Source: CAD feature listing. Evaluate the final solid. Frame: model axes, mm. Face numbers are marked on the shaded views. A direction names the side the tool comes from. Give positions to 0.01 mm unless a question says otherwise; leave off trailing zeros. Write each loop counter-clockwise with the first axis right and the second up, starting at its lowest first coordinate (ties: lowest second). Pieces come first, ordered by that corner, then holes. Notation, with made-up numbers: M 84.25,47.5 L 128.25,47.5 A15 ccw 128.25,71.5 Z; hole C -18.75,24 d11. An arc over 180 degrees is marked long. Return JSON: item names as keys, results as strings.
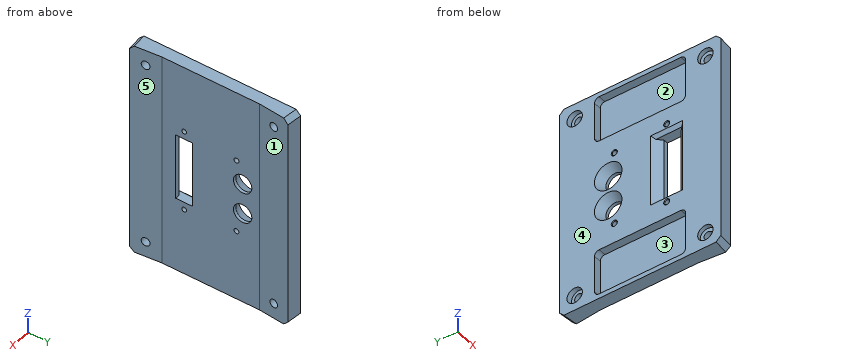
```python
from build123d import *

# Parameters (mm, degrees)
SKETCH021_W      = 59.427886
SKETCH021_H      = 30
PAD012_DEPTH     = 5
FILLET003_R      = 3
PAD011_DEPTH     = 70
SKETCH017_R      = 2.7
POCKET006_DEPTH  = 12
SKETCH018_R      = 5
POCKET007_DEPTH  = 5
CHAMFER008_SIZE  = 3
SKETCH019_R      = 1.55
SKETCH019_W      = 11
SKETCH019_H      = 43
POCKET008_DEPTH  = 20
CHAMFER009_SIZE  = 5
CHAMFER010_SIZE  = 2
SKETCH020_R      = 1.6
SKETCH020_R_2    = 6
POCKET009_DEPTH  = 14
CHAMFER011_SIZE2 = 6
CHAMFER011_SIZE  = 3
CHAMFER012_SIZE  = 0.4


with BuildPart() as obj1:
    # Sketch021 (on Face1 of CopyChamfer012) → Pad012 (new body)
    with BuildSketch(Plane(origin=(-79.911931, 0, 0), x_dir=(0, -1, 0), z_dir=(-1, 0, 0))):
        with Locations((0, 52)):
            Rectangle(SKETCH021_W, SKETCH021_H)
    extrude(amount=-PAD012_DEPTH)

    # Mirrored007: obj1 across XY


with BuildPart() as obj1_1:
    add(obj1.part)
    add(obj1.part.mirror(Plane.XY))

    # Fillet003
    fillet003_edges = [obj1_1.edges().sort_by_distance(p)[0] for p in [
        (-77.411931, -29.713943, 67),
        (-77.411931, -29.713943, 37),
        (-77.411931, 29.713943, 67),
        (-77.411931, 29.713943, -37),
        (-77.411931, -29.713943, -37),
        (-77.411931, 29.713943, 37),
        (-77.411931, 29.713943, -67),
        (-77.411931, -29.713943, -67),
    ]]
    fillet(fillet003_edges, radius=FILLET003_R)


with BuildPart() as cut:
    # Sketch016 (on XY_Plane010 of Origin020) → Pad011 (new body, symmetric)
    with BuildSketch(Plane.XY):
        Polygon((-70.037094, -51.784164), (-71.911931, -31.872233), (-71.911931, 31.872233), (-70.037094, 51.784164), (-79.911931, 52.713943), (-79.911931, -52.713943), align=None)
    extrude(amount=PAD011_DEPTH, both=True)

    # Sketch017 (on Face1 of Pad011) → Pocket006 (cut)
    with BuildSketch(Plane(origin=(-74.254608, -6.991552, 0), x_dir=(-0.093742, 0.995597, 0), z_dir=(0.995597, 0.093742, 0))):
        with Locations((-34.990726, 60)):
            Circle(SKETCH017_R)
        with Locations((-34.990726, -60)):
            Circle(SKETCH017_R)
    pocket006 = extrude(amount=-POCKET006_DEPTH, mode=Mode.SUBTRACT)

    # Sketch018 (on Face1 of Pocket006) → Pocket007 (cut)
    with BuildSketch(Plane(origin=(-80.228187, -7.554003, 0), x_dir=(-0.093742, 0.995597, 0), z_dir=(0.995597, 0.093742, 0))):
        with Locations((-34.990726, 60)):
            Circle(SKETCH018_R)
        with Locations((-34.990726, -60)):
            Circle(SKETCH018_R)
    pocket007 = extrude(amount=-POCKET007_DEPTH, mode=Mode.SUBTRACT)

    # Mirrored006: Pocket006, Pocket007 across XZ
    add(pocket006.mirror(Plane.XZ), mode=Mode.SUBTRACT)
    add(pocket007.mirror(Plane.XZ), mode=Mode.SUBTRACT)

    # Chamfer008
    chamfer008_edges = [cut.edges().sort_by_distance(p)[0] for p in [
        (-74.974512, 52.249054, 70),
        (-74.974512, 52.249054, -70),
        (-74.974512, -52.249054, 70),
        (-74.974512, -52.249054, -70),
    ]]
    chamfer(chamfer008_edges, length=CHAMFER008_SIZE)

    # Sketch019 (on Face7 of Chamfer008) → Pocket008 (cut)
    with BuildSketch(Plane.YZ.offset(-71.911931)):
        with Locations((-17.372233, 26.5)):
            Circle(SKETCH019_R)
        with Locations((-17.372233, -26.5)):
            Circle(SKETCH019_R)
        with Locations((-17.372233, 0)):
            Rectangle(SKETCH019_W, SKETCH019_H)
    extrude(amount=-POCKET008_DEPTH, mode=Mode.SUBTRACT)

    # Chamfer009
    chamfer009_edges = [cut.edges().sort_by_distance(p)[0] for p in [
        (-79.911931, -11.872233, 0),
        (-79.911931, -22.872233, 0),
    ]]
    chamfer(chamfer009_edges, length=CHAMFER009_SIZE)

    # Chamfer010
    chamfer010_edges = [cut.edges().sort_by_distance(p)[0] for p in [
        (-79.911931, -17.372233, 21.5),
        (-79.911931, -17.372233, -21.5),
    ]]
    chamfer(chamfer010_edges, length=CHAMFER010_SIZE)

    # Sketch020 (on Face24 of Chamfer010) → Pocket009 (cut)
    with BuildSketch(Plane.YZ.offset(-71.911931)):
        with Locations((16.8, 24)):
            Circle(SKETCH020_R)
        with Locations((16.8, -24)):
            Circle(SKETCH020_R)
        with Locations((20.8, 10)):
            Circle(SKETCH020_R_2)
        with Locations((20.8, -10)):
            Circle(SKETCH020_R_2)
    extrude(amount=-POCKET009_DEPTH, mode=Mode.SUBTRACT)

    # Chamfer011
    chamfer011_edges = [cut.edges().sort_by_distance(p)[0] for p in [
        (-79.911931, 14.8, 10),
        (-79.911931, 14.8, -10),
    ]]
    chamfer011_side = cut.faces().sort_by_distance((-79.911931, 0.943229, 0))[0]
    chamfer(chamfer011_edges, length=CHAMFER011_SIZE, length2=CHAMFER011_SIZE2, reference=chamfer011_side)

    # Chamfer012
    chamfer012_edges = [cut.edges().sort_by_distance(p)[0] for p in [
        (-79.911931, 15.2, -24),
        (-79.911931, 15.2, 24),
        (-79.911931, -18.922233, 26.5),
        (-79.911931, -18.922233, -26.5),
    ]]
    chamfer(chamfer012_edges, length=CHAMFER012_SIZE)

    # Cut: cut obj1
    add(obj1_1.part, mode=Mode.SUBTRACT)


solid = cut.part
```
1) Contact query for flat-ended pins moving along their axis: pin 1 Ø2 at (x, z) = (-74, -1.5) entering from -Y; pin 2 Ø2.5 at (y, z) = (16.8, -24) entering from +X; pin 3 Ø6 at (y, z) = (6, 43.5) entering from +X; pin 4 Ø0.9 at (x, z) = (-73, 8) entering from +Y. Output: stop coordinate, or through.
Numbers:
{"pin 1": "stops at y = -52.25", "pin 2": "passes through", "pin 3": "stops at x = -71.91", "pin 4": "stops at y = 52.11"}
2) Cut plane C-C, the plane y = 1. Return the cut outline in (x, z).
Numbers:
{"outline": "M -79.91,-70 L -71.91,-70 L -71.91,70 L -79.91,70 L -79.91,67 L -74.91,67 L -74.91,37 L -79.91,37 L -79.91,-37 L -74.91,-37 L -74.91,-67 L -79.91,-67 Z"}
3) Cut plane D-D, the plane z = -48.5. Return the cut outline in (x, y).
Numbers:
{"outline": "M -79.91,-52.71 L -70.04,-51.78 L -71.91,-31.87 L -71.91,31.87 L -70.04,51.78 L -79.91,52.71 L -79.91,29.71 L -74.91,29.71 L -74.91,-29.71 L -79.91,-29.71 Z"}
4) Set-up query: the marked faces 1 and 2. Return all of +Z, -Z, +X, -X, +Y, -Y with unobstructed straight access to the full face (end or side cutting, diameter ignored); none if empty.
Numbers:
{"face 1": "+Z, -Z, +X", "face 2": "-X"}
5) Line query: line 1 (Z direction, x = -73.25, y = 20.8); line 2 (Z direction, x = -78.25, y = -7); line 3 (Z direction, x = -74.25, y = -12.5). Output: solid intervals per line, ascending. Write a range as [from, to].
Numbers:
{"line 1": "z = [-70, -16], [-4, 4], [16, 70]", "line 2": "z = [-70, -67], [-37, 37], [67, 70]", "line 3": "z = [-70, -21.5], [21.5, 70]"}
6) Cut plane B-B, the plane z = 10. Return the cut outline in (x, y), then the cut area to 3 significant figures.
Numbers:
{"outline": "M -79.91,-52.71 L -70.04,-51.78 L -71.91,-31.87 L -71.91,-22.87 L -74.91,-22.87 L -79.91,-27.87 Z; M -79.91,-6.87 L -74.91,-11.87 L -71.91,-11.87 L -71.91,14.8 L -73.91,14.8 L -79.91,11.8 Z; M -79.91,29.8 L -73.91,26.8 L -71.91,26.8 L -71.91,31.87 L -70.04,51.78 L -79.91,52.71 Z", "area": "648 mm²"}
7) Cut plane A-A, the plane y = 20.8. Return the cut outline in (x, z), then the cut area to 3 significant figures.
Numbers:
{"outline": "M -79.91,-70 L -71.91,-70 L -71.91,-16 L -73.91,-16 L -79.91,-19 L -79.91,-37 L -74.91,-37 L -74.91,-67 L -79.91,-67 Z; M -79.91,-1 L -73.91,-4 L -71.91,-4 L -71.91,4 L -73.91,4 L -79.91,1 Z; M -79.91,19 L -73.91,16 L -71.91,16 L -71.91,70 L -79.91,70 L -79.91,67 L -74.91,67 L -74.91,37 L -79.91,37 Z", "area": "592 mm²"}
8) Draft query along Y for the marked faces 3, 4 and 5. Return one class per face: released by +Y, released by -Y, zero draft, split by the parting line, or undercut.
Numbers:
{"face 3": "undercut", "face 4": "zero draft", "face 5": "undercut"}
